The listing builds one solid part. Answer for the finished solid, in the listing's coordinates (mm). Face numbers are marked on the shaded views. A direction names the side the tool comes from. Give positions to 0.01 mm unless a question says otherwise; leave off trailing zeros. Order: outer loops, then holes, each group sorted by start corner. A loop starts at its lowest first (then second) coordinate and runs counter-clockwise, first axis right, second up.
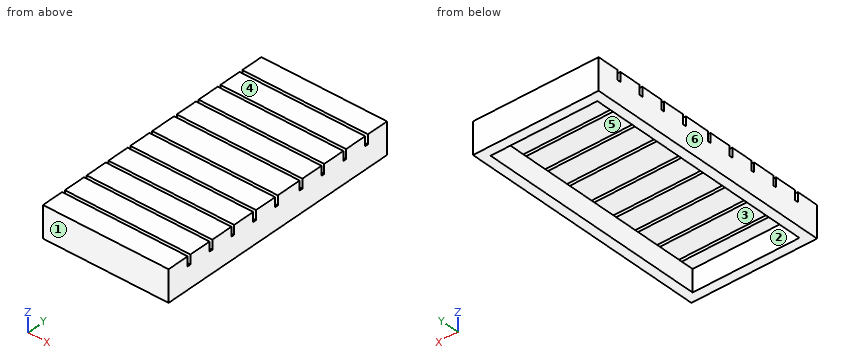
```python
from build123d import *

# Parameters (mm, degrees)
F0_W     = 508
F0_H     = 1016
F1_DEPTH = 88.9
F2_W     = 431.8
F2_H     = 939.8
F6_DEPTH = 88.9
F3_W     = 508
F3_H     = 1016
F4_DEPTH = 38.1
F5_W     = 508
F5_H     = 12.7
F7_DEPTH = 38.1


with BuildPart() as f1:
    # F0 (on Top) → F1 (new body)
    with BuildSketch(Plane.XY):
        Rectangle(F0_W, F0_H)
    extrude(amount=F1_DEPTH)

    # F2 (on face) → F6 (cut)
    with BuildSketch(Plane(origin=(0, 0, 0), x_dir=(1, 0, 0), z_dir=(0, 0, -1))):
        Rectangle(F2_W, F2_H)
    extrude(amount=-F6_DEPTH, mode=Mode.SUBTRACT)

    # F3 (on face) → F4 (join)
    with BuildSketch(Plane.XY.offset(88.9)):
        Rectangle(F3_W, F3_H)
    extrude(amount=F4_DEPTH)

    # F5 (on face) → F7 (cut)
    with BuildSketch(Plane.XY.offset(127)):
        with Locations((0, 412.75)):
            Rectangle(F5_W, F5_H)
        with Locations((0, 311.15)):
            Rectangle(F5_W, F5_H)
        with Locations((0, 209.55)):
            Rectangle(F5_W, F5_H)
        with Locations((0, 107.95)):
            Rectangle(F5_W, F5_H)
        with Locations((0, -6.35)):
            Rectangle(F5_W, F5_H)
        with Locations((0, -107.95)):
            Rectangle(F5_W, F5_H)
        with Locations((0, -209.55)):
            Rectangle(F5_W, F5_H)
        with Locations((0, -311.15)):
            Rectangle(F5_W, F5_H)
        with Locations((0, -412.75)):
            Rectangle(F5_W, F5_H)
    extrude(amount=-F7_DEPTH, mode=Mode.SUBTRACT)


solid = f1.part
```
1) For a pull along X with two mould halves and no side action, classify the marked faces 3, 4, 5 and 6 as +X half, -X half, draft (parallel to the pull), parting line (faces both ways), or undercut.
Geometry says:
face 3: undercut
face 4: draft
face 5: undercut
face 6: -X half
2) Find section C-C (z = 111). Count the separate pieces of the cut face and the enclosed holes in it, then the cut area to 3 significant figures.
Geometry says:
separate pieces: 10
enclosed holes: 0
area: 458,000 mm2
3) Given P1, Ø14, axis at x = 240, y = 411, coming from the +Z side; P2, Ø1, axis at x = -199.5, y = -391, coming from the -Z side; P3, Ø4, axis at x = 238.5, y = -312, coming from the +Z side, each flat-ended and moving along its own axis, determine where each tip first touches the part or whether it passes through.
Geometry says:
P1: stops at z = 127
P2: stops at z = 88.9
P3: stops at z = 88.9
4) A tool of negligible diameter and unlimited length cuts with its end or side. For the marked faces 1 and 2, from which of +Z, -Z, +X, -X, +Y, -Y can it reach the whole face along a straight path? Write none if from no direction.
Geometry says:
face 1: +Z, -Z, +X, -X, -Y
face 2: -Z
5) Straight lines are drawn through the part: probe 1 along X at (y, z) = (27, 61.5); probe 2 along Y at (x, z) = (-54, 19); probe 3 along Z at (x, y) = (-63.5, 434). For each, find the intervals that lie inside material, in ascending order.
Geometry says:
probe 1: x = -254 to -215.9, 215.9 to 254
probe 2: y = -508 to -469.9, 469.9 to 508
probe 3: z = 88.9 to 127
6) Find section A-A (y = 350). Write down the section's boundary in (x, z).
Geometry says:
outline: (-254, 0) - (-215.9, 0) - (-215.9, 88.9) - (215.9, 88.9) - (215.9, 0) - (254, 0) - (254, 127) - (-254, 127) - close
7) Find section B-B (z = 63). Write down the section's boundary in (x, y), then the cut area to 3 significant figures.
Geometry says:
outline: (-254, -508) - (254, -508) - (254, 508) - (-254, 508) - close; hole (-215.9, -469.9) - (215.9, -469.9) - (215.9, 469.9) - (-215.9, 469.9) - close
area: 110,000 mm2
